Geometry check sheet. Reference: the model listing, model coordinates, mm. A direction names the side the tool comes from. Give positions to 0.01 mm unless a question says otherwise; leave off trailing zeros. Order: outer loops, then holes, each group sorted by start corner. A loop starts at its lowest first (then second) coordinate and runs counter-clockwise, first axis right, second up. Notation, with made-up numbers: (-17.75, -1) - (4.25, -1) arc R16 ccw to (4.25, 19) - close; hole circle Ø10 at (-18, -12). An arc over 180 degrees is marked (long way). Put each result on its own line as item: value. Start each with the question number.
```python
from build123d import *

# Parameters (mm, degrees)
SKETCH1_R            = 24.505905818
BOSS_EXTRUDE1_DEPTH  = 0.2286
BOSS_EXTRUDE2_START  = 63.5
BOSS_EXTRUDE2_DEPTH  = 63.5
SKETCH4_W            = 63.5
SKETCH4_H            = 76.2
BOSS_EXTRUDE4_DEPTH  = 14.929782549
SKETCH5_W            = 63.5
SKETCH5_H            = 50.8
BOSS_EXTRUDE5_DEPTH  = 44.789347647
FILLET2_R            = 25.4
SKETCH7_W            = 63.5
SKETCH7_H            = 25.4
BOSS_EXTRUDE7_DEPTH  = 22.41804
FILLET2_OF_MIRROR1_R = 25.4
SKETCH10_W           = 48.26
SKETCH10_H           = 64.77
CUT_EXTRUDE2_DEPTH   = 179.030869421
FILLET3_R            = 7.62


# Some blends are built 0.0001 mm under size
with BuildPart() as part:
    # Sketch1 → Boss-Extrude1 (new body)
    with BuildSketch(Plane.YZ):
        with Locations(Location((0, 0, 0), (0, 0, 270))):
            Circle(SKETCH1_R)
    extrude(amount=BOSS_EXTRUDE1_DEPTH)

    # Sketch2 → Boss-Extrude2 (add)
    with BuildSketch(Plane(origin=(0, 0, 0), x_dir=(0, -1, 0), z_dir=(-1, 0, 0)).offset(BOSS_EXTRUDE2_START)):
        with BuildLine():
            Line((-24.505905818, 0), (-24.505905818, 76.2))
            Line((-24.505905818, 76.2), (24.505905818, 76.2))
            Line((24.505905818, 76.2), (24.505905818, 0))
            ThreePointArc((24.505905818, 0), (0, -24.505905818), (-24.505905818, 0))
        make_face()
    extrude(amount=-BOSS_EXTRUDE2_DEPTH)

    # Sketch4 → Boss-Extrude4 (add)
    with BuildSketch(Plane.XY.offset(76.2)):
        with Locations((-31.75, 0)):
            Rectangle(SKETCH4_W, SKETCH4_H)
    extrude(amount=BOSS_EXTRUDE4_DEPTH)

    # Sketch5 → Boss-Extrude5 (add)
    with BuildSketch(Plane(origin=(0, 38.1, 0), x_dir=(-1, 0, 0), z_dir=(0, 1, 0))):
        with Locations((31.75, 101.6)):
            Rectangle(SKETCH5_W, SKETCH5_H)
    boss_extrude5 = extrude(amount=BOSS_EXTRUDE5_DEPTH)

    # Fillet2
    fillet2_edges = [part.edges().sort_by_distance(p)[0] for p in [
        (-31.75, 82.889347647, 76.2),
        (-31.75, 82.889347647, 127),
    ]]
    fillet(fillet2_edges, radius=FILLET2_R - 0.0001)  # a hair under: the kernel refuses the full size

    # Sketch7 → Boss-Extrude7 (add)
    with BuildSketch(Plane.XZ.offset(-38.1)):
        with Locations((-31.75, 114.3)):
            Rectangle(SKETCH7_W, SKETCH7_H)
    boss_extrude7 = extrude(amount=BOSS_EXTRUDE7_DEPTH)

    # Mirror1: Boss-Extrude5, Boss-Extrude7 across plane
    add(boss_extrude5.mirror(Plane.ZX))
    add(boss_extrude7.mirror(Plane.ZX))

    # Fillet2 of Mirror1
    fillet2_of_mirror1_edges = [part.edges().sort_by_distance(p)[0] for p in [
        (-31.75, -82.889347647, 76.2),
        (-31.75, -82.889347647, 127),
    ]]
    fillet(fillet2_of_mirror1_edges, radius=FILLET2_OF_MIRROR1_R - 0.0001)  # a hair under: the kernel refuses the full size

    # Sketch10 → Cut-Extrude2 (cut, through all)
    with BuildSketch(Plane(origin=(0, 24.505905818, 0), x_dir=(-1, 0, 0), z_dir=(0, 1, 0))):
        with Locations((31.75, 34.925)):
            Rectangle(SKETCH10_W, SKETCH10_H)
    extrude(amount=-CUT_EXTRUDE2_DEPTH, mode=Mode.SUBTRACT)

    # Fillet3
    # the kernel refuses this fillet: 7.62 mm, written as the material it takes off along each edge
    with BuildSketch(Plane(origin=(-7.62, -24.505905818, 2.54), x_dir=(0, 0.11378574923272014, -0.9935053111441069), z_dir=(-1, 0, 0))) as fillet3_piece_1:
        with BuildLine():
            CenterArc((8.526567897, -7.480642321), FILLET3_R, 79.025374556, 107.50821933)
            Line((0.956057426, -8.34768973), (0.199006379, -8.434394471))
            Line((0.199006379, -8.434394471), (-0.757051047, -0.086704741))
            Line((-0.757051047, -0.086704741), (-0.086704741, 0.757051047))
            ThreePointArc((-0.086704741, 0.757051047), (2.436798749, 1.04606685), (10.122284809, 0.748064232))
            Line((10.122284809, 0.748064232), (9.977219635, 0))
        make_face()
    extrude(amount=48.26, mode=Mode.SUBTRACT)
    with BuildSketch(Plane(origin=(-7.62, 24.505905818, 2.54), x_dir=(0, -0.11378574923272022, -0.9935053111441069), z_dir=(-1, 0, 0))) as fillet3_piece_2:
        with BuildLine():
            CenterArc((8.526567897, 7.480642321), FILLET3_R, 173.466406113, 107.50821933)
            Line((0.956057426, 8.34768973), (0.199006379, 8.434394471))
            Line((0.199006379, 8.434394471), (-0.757051047, 0.086704741))
            Line((-0.757051047, 0.086704741), (-0.086704741, -0.757051047))
            ThreePointArc((-0.086704741, -0.757051047), (2.436798749, -1.04606685), (10.122284809, -0.748064232))
            Line((10.122284809, -0.748064232), (9.977219635, 0))
        make_face()
    extrude(amount=48.26, mode=Mode.SUBTRACT)


solid = part.part
```
Item 1: Cross-section at B-B (z = 43.5). Enter the section's corners in (x, y).
Item 2: Thickness scan on line 1 along Z through (x, y) = (-17.5, -30); line 2 along X through (y, z) = (-0.5, 51); line 3 along Z through (x, y) = (-32, -19.5). Record the ranges inside material, lowest first.
Item 3: Set-up check for faces 4 (the face through (-32, 27, 101.6)), 5 (the face through (-31.41, -22.31, -0.66)), 6 (the face through (-31.412, 22.189, -0.494)): record each of +Z, -Z, +X, -X, +Y, -Y from which the full face is reachable in a straight line by a thin tool's end or side.
Item 4: Cross-section at A-A (y = -27). Enter the section's corners in (x, z).
Item 5: Cross-section at C-C (y = 0). Enter the section's corners in (x, z), and give its area (3 significant figures).
Item 6: Release check for a two-part mould opening along Y. For faces 1 (the face through (-30, 24.506, 69)), 2 (the face through (-31, 38.1, 96)), 3 (the face through (-31, 0, 67.31)) record: +Y half, -Y half, draft (parallel to the pull), parting line (faces both ways), or undercut.
Item 7: Gauge pin test, flat ends, axial feed: pin 1 Ø6.5 at (x, y) = (-16.5, 29.5) entering from -Z; pin 2 Ø24.5 at (x, y) = (-33, -22.5) entering from -Z; pin 3 Ø19 at (x, y) = (-47.5, -14) entering from +Z; pin 4 Ø8.5 at (x, z) = (-46, 97) entering from +Y. Record the tip position at first contact, or that the pin passes through.
Recorded:
1. outline: (-63.5, -24.51) - (-55.88, -24.51) - (-55.88, 24.51) - (-63.5, 24.51) - close; (-7.62, -24.51) - (0, -24.51) - (0, 24.51) - (-7.62, 24.51) - close
2. line 1: z = 76.2 to 91.13, 101.6 to 127
2. line 2: x = -63.5 to -55.88, -7.62 to 0
2. line 3: z = -14.84 to 1.74, 67.31 to 91.13, 101.6 to 127
3. face 4: +X, -X
3. face 5: -Y
3. face 6: +Y
4. outline: (-63.5, 76.2) - (0, 76.2) - (0, 91.13) - (-63.5, 91.13) - close; (-63.5, 101.6) - (0, 101.6) - (0, 127) - (-63.5, 127) - close
5. outline: (-63.5, -24.51) - (0.23, -24.51) - (0.23, 24.51) - (0, 24.51) - (0, 91.13) - (-63.5, 91.13) - close; hole (-55.88, 2.54) - (-7.62, 2.54) - (-7.62, 67.31) - (-55.88, 67.31) - close
5. area: 4,230 mm^2
6. face 1: +Y half
6. face 2: undercut
6. face 3: draft
7. pin 1: stops at z = 76.2
7. pin 2: stops at z = -22.26
7. pin 3: stops at z = 127
7. pin 4: stops at y = 82.89
